```python
from build123d import *

# Parameters (mm, degrees)
EXTRUDE048_DEPTH = 0.8
EXTRUDE047_DEPTH = 2
FILLET_R         = 0.5


with BuildPart() as extrude_switch_hole:
    # Sketch047 → Extrude048 (new body, symmetric)
    with BuildSketch(Plane.XZ):
        Polygon((0, 0.8), (3, 0.8), (3, -0.8), (0, -0.8), (0, 0), align=None)
    extrude(amount=EXTRUDE048_DEPTH, both=True)


with BuildPart() as cut_toggle_switch_cover:
    # Sketch046 → Extrude047 (new body, symmetric)
    with BuildSketch(Plane.XZ):
        with BuildLine():
            add(Edge.make_bspline(
                [(0, 6), (2, 4), (4, 4)],
                knots=[0, 0, 0, 1, 1, 1], degree=2))
            Line((0, 6), (0, 0))
            Line((0, 0), (0, -6))
            add(Edge.make_bspline(
                [(4, -4), (2, -4), (0, -6)],
                knots=[0, 0, 0, 1, 1, 1], degree=2))
            Line((4, -4), (4, 0))
            Line((4, 0), (4, 4))
        make_face()
    extrude(amount=EXTRUDE047_DEPTH, both=True)

    # Fillet
    fillet_edges = [cut_toggle_switch_cover.edges().sort_by_distance(p)[0] for p in [
        (4, 0, 4),
        (4, 0, -4),
        (4, 2, -2),
        (4, -2, -2),
        (4, 2, 2),
        (4, -2, 2),
    ]]
    fillet(fillet_edges, radius=FILLET_R)

    # Cut012: cut Extrude_Switch_hole
    add(extrude_switch_hole.part, mode=Mode.SUBTRACT)


solid = cut_toggle_switch_cover.part
```
Design review of the part built by this model. Coordinates are the model's own, in mm. A direction names the side the tool comes from. Coordinates: 2 decimals unless noted, no trailing zeros. Loops run counter-clockwise (first coordinate to the right, second up) from the corner with the lowest first, then second, coordinate; pieces in that order, holes last. Notation, with made-up numbers: (74.25, -2) - (98.25, -2) arc R25 ccw to (98.25, 33) - close; hole circle Ø5 at (29.5, -38). An arc over 180 degrees is marked (long way). Use CSV: the item, a comma, the result in double quotes. Start each with the question number.
1) For pin 1 Ø0.5 at (x, y) = (1.5, 0.5) entering from -Z; pin 2 Ø0.5 at (x, y) = (1.5, 0) entering from +Z; pin 3 Ø2 at (y, z) = (-1.5, -4.5) entering from +X, all flat-tipped, find the tip position at first contact; note any pin that passes through.
2) Wall thickness on L1, parallel to X at y = -0.95, z = -4.5; L2, parallel to Y at x = 2.35, z = -0.5; L3, parallel to X at y = -0.1, z = 0.5: over which ranges is each line inside the solid? List them lowest first. Write a range as from..to.
3) Tool access review of faces 1 (the flat face through (0, -1, 0)), 2 (the flat face through (2, 0.8, 0)): name each direction out of +Z, -Z, +X, -X, +Y, -Y from which nothing blocks a thin tool from reaching the whole face with its end or side.
4) The part is to be moulded in two halves that separate along Y. For faces 3 (the flat face through (2, -2, 0)), 4 (the flat face through (1, 0, 0.8)), 5 (the flat face through (2, -0.8, 0)), 6 (the flat face through (2, 2, 0)), say which applies: +Y half, -Y half, draft (parallel to the pull), parting line (faces both ways), or undercut.
5) Consider section A-A on z = -0.5. Write out the cut boundary in (x, y).
Geometry says:
1,pin 1,"z = -4.95"
1,pin 2,"z = 4.95"
1,pin 3,"x = 4"
2,L1,"0..2"
2,L2,"-2..-0.8, 0.8..2"
2,L3,"3..4"
3,face 1,"+Z, -Z, -X, +Y, -Y"
3,face 2,"-X"
4,face 3,"-Y half"
4,face 4,"undercut"
4,face 5,"undercut"
4,face 6,"+Y half"
5,outline,"(0, -2) - (3.5, -2) arc R0.5 ccw to (4, -1.5) - (4, 1.5) arc R0.5 ccw to (3.5, 2) - (0, 2) - (0, 0.8) - (3, 0.8) - (3, -0.8) - (0, -0.8) - close"
